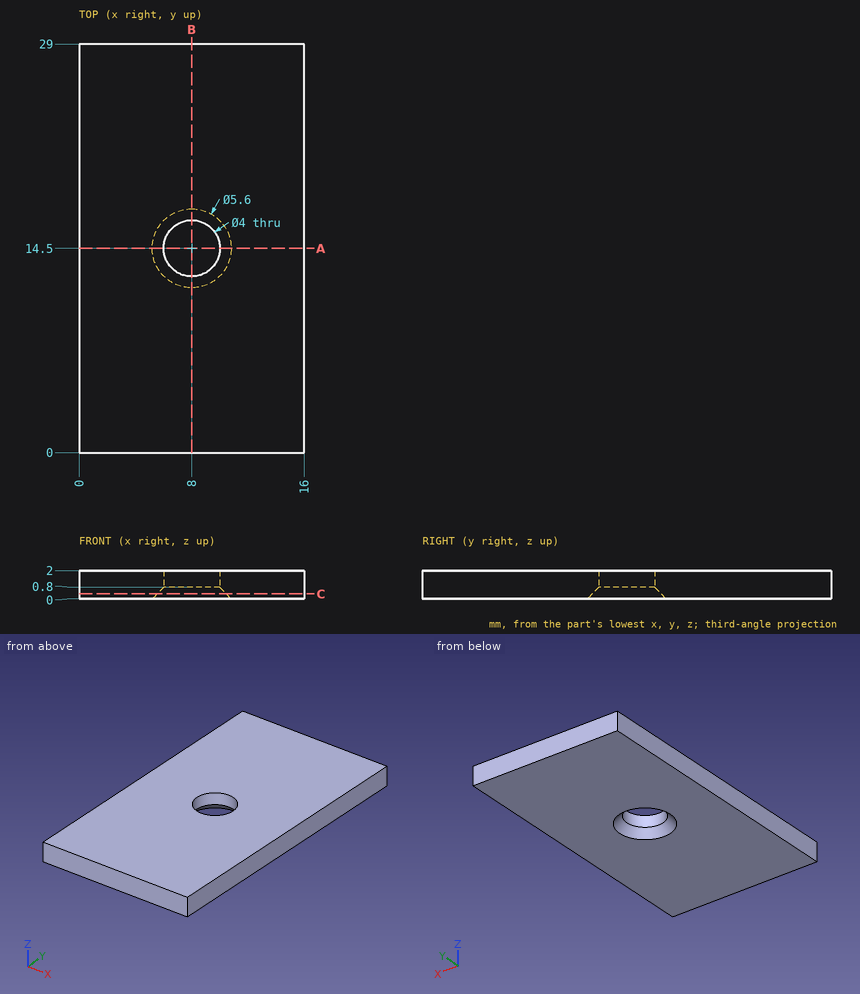
Print and shaded views of the part. All mm, measured from the part's lowest x, y and z. Round coordinates to 2 decimals unless told otherwise and drop trailing zeros. Write each loop counter-clockwise with the first axis right and the second up, starting at its lowest first coordinate (ties: lowest second). Pieces come first, ordered by that corner, then holes. Notation, with made-up numbers: (80.5, -13) -> (90.5, -13) arc R20 ccw to (90.5, 22) -> close; hole circle Ø4 at (-38, -33.5). An arc over 180 degrees is marked (long way). Return JSON: item names as keys, results as strings. Group by question number.
Q1. Saw through at C-C on z = 0.35. Write the cut outline in (x, y).
Q2. Saw through at A-A on y = 14.5. Write the cut outline in (x, z).
Q3. Probe L1, parallel to X at y = 14.5, z = 1.15; L2, parallel to Y at x = 7.25, z = 1.8; L3, parallel to Y at x = 9.5, z = 0.45. List the from-to ranges inside material, lowest first. Write a range as [from, to].
Q4. Saw through at B-B on x = 8. Write the cut outline in (y, z).
Q5. Pin check, flat tips, straight feed: pin 1 (1.5 mm diameter, centred on x = 12, y = 5.5, fed in from -Z); pin 2 (5 mm diameter, centred on x = 8, y = 14.5, fed in from -Z). Stop position of each tip, or through.
Answer:
{
 "1": {"outline": "(0, 0) -> (16, 0) -> (16, 29) -> (0, 29) -> close; hole circle Ø4.9 at (8, 14.5)"},
 "2": {"outline": "(0, 0) -> (5.2, 0) -> (6, 0.8) -> (6, 2) -> (0, 2) -> close; (10, 0.8) -> (10.8, 0) -> (16, 0) -> (16, 2) -> (10, 2) -> close"},
 "3": {"L1": "[0, 6], [10, 16]", "L2": "[0, 12.65], [16.35, 29]", "L3": "[0, 12.69], [16.31, 29]"},
 "4": {"outline": "(0, 0) -> (11.7, 0) -> (12.5, 0.8) -> (12.5, 2) -> (0, 2) -> close; (16.5, 0.8) -> (17.3, 0) -> (29, 0) -> (29, 2) -> (16.5, 2) -> close"},
 "5": {"pin 1": "z = 0", "pin 2": "z = 0.3"}
}
